```python
from build123d import *

# Parameters (mm, degrees)
SKETCH1_W           = 152.4
SKETCH1_H           = 68.072
BOSS_EXTRUDE1_DEPTH = 2.3622
SKETCH2_W           = 26.67
SKETCH2_H           = 13.97
SKETCH2_W_2         = 23.622
CUT_EXTRUDE1_DEPTH  = 167.92853912
FILLET1_R           = 3.81
SKETCH4_W           = 68.072
SKETCH4_H           = 2.3622
BOSS_EXTRUDE2_DEPTH = 101.6
SKETCH5_R           = 3.2639
CUT_EXTRUDE2_DEPTH  = 167.92853912


with BuildPart() as part:
    # Sketch1 → Boss-Extrude1 (new body)
    with BuildSketch(Plane(origin=(0, 0, 0), x_dir=(1, 0, 0), z_dir=(0, 1, 0))):
        with Locations((76.2, 34.036)):
            Rectangle(SKETCH1_W, SKETCH1_H)
    extrude(amount=BOSS_EXTRUDE1_DEPTH)

    # Sketch2 → Cut-Extrude1 (cut, through all)
    with BuildSketch(Plane(origin=(0, 2.3622, 0), x_dir=(1, 0, 0), z_dir=(0, 1, 0))):
        with Locations((43.815, 47.371)):
            Rectangle(SKETCH2_W, SKETCH2_H)
        with Locations((95.631, 47.371)):
            Rectangle(SKETCH2_W_2, SKETCH2_H)
        with Locations((43.815, 20.701)):
            Rectangle(SKETCH2_W, SKETCH2_H)
        with Locations((95.631, 20.701)):
            Rectangle(SKETCH2_W_2, SKETCH2_H)
    extrude(amount=-CUT_EXTRUDE1_DEPTH, mode=Mode.SUBTRACT)

    # Fillet1
    fillet1_edges = [part.edges().sort_by_distance(p)[0] for p in [
        (83.82, 1.1811, -40.386),
        (83.82, 1.1811, -54.356),
        (107.442, 1.1811, -54.356),
        (107.442, 1.1811, -40.386),
        (30.48, 1.1811, -13.716),
        (30.48, 1.1811, -27.686),
        (57.15, 1.1811, -27.686),
        (57.15, 1.1811, -13.716),
        (83.82, 1.1811, -13.716),
        (83.82, 1.1811, -27.686),
        (107.442, 1.1811, -27.686),
        (107.442, 1.1811, -13.716),
        (30.48, 1.1811, -40.386),
        (30.48, 1.1811, -54.356),
        (57.15, 1.1811, -54.356),
        (57.15, 1.1811, -40.386),
    ]]
    fillet(fillet1_edges, radius=FILLET1_R)

    # Sketch4 → Boss-Extrude2 (add)
    with BuildSketch(Plane.ZY):
        with Locations((-34.036, 1.1811)):
            Rectangle(SKETCH4_W, SKETCH4_H)
    extrude(amount=BOSS_EXTRUDE2_DEPTH)

    # Sketch5 → Cut-Extrude2 (cut, through all)
    with BuildSketch(Plane.XZ):
        with Locations(Location((139.7, -12.446, 0), (0, 0, 270))):
            Circle(SKETCH5_R)
        with Locations(Location((139.7, -55.626, 0), (0, 0, 270))):
            Circle(SKETCH5_R)
    extrude(amount=-CUT_EXTRUDE2_DEPTH, mode=Mode.SUBTRACT)


solid = part.part
```
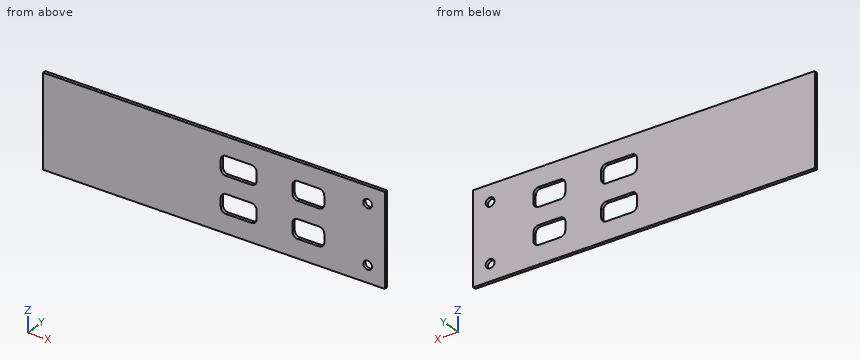
Input: part model. Units: mm. Frame: model coordinates. Give positions to 0.01 mm unless a question says otherwise; leave off trailing zeros. Loops run counter-clockwise (first coordinate to the right, second up) from the corner with the lowest first, then second, coordinate; pieces in that order, holes last. Notation, with made-up numbers: (54.25, -21.5) -> (81.25, -21.5) arc R12 cw to (81.25, -15.5) -> close; hole circle Ø9 at (-9.5, 66). An arc over 180 degrees is marked (long way). Use a Markdown table: item, result.
Q1. First-contact query: P1, Ø3, axis at x = 104, z = -18.5, coming from the +Y side. Flat tip, straight axial feed; report the tip coordinate or a pass-through.
Entries:
| item | result |
|---|---|
| P1 | passes through |
Q2. Ray query, probe 1 along X at (y, z) = (1.3, -47); probe 2 along Z at (x, y) = (44.5, 2.25); probe 3 along Z at (x, y) = (104, 1). Return the intervals inside material, ascending. Write a range as from..to.
Entries:
| item | result |
|---|---|
| probe 1 | x = -101.6..30.48, 57.15..83.82, 107.44..152.4 |
| probe 2 | z = -68.07..-54.36, -40.39..-27.69, -13.72..0 |
| probe 3 | z = -68.07..-54.34, -40.4..-27.67, -13.73..0 |
Q3. Section query A-A, the plane x = 139.7. Return the cut outline in (y, z), plus the area to 3 significant figures.
Entries:
| item | result |
|---|---|
| outline | (0, -68.07) -> (2.36, -68.07) -> (2.36, -58.89) -> (0, -58.89) -> close; (0, -52.36) -> (2.36, -52.36) -> (2.36, -15.71) -> (0, -15.71) -> close; (0, -9.18) -> (2.36, -9.18) -> (2.36, 0) -> (0, 0) -> close |
| area | 130 mm² |
Q4. Section query B-B, the plane y = 1.95. State how many separate pieces and enclosed holes the cut face has, plus the area to 3 significant figures.
Entries:
| item | result |
|---|---|
| separate pieces | 1 |
| enclosed holes | 6 |
| area | 15,900 mm² |
